```python
from build123d import *

# Parameters (mm, degrees)
F1_DEPTH = 5.08
F2_R     = 5.334
F2_R_2   = 2.54
F3_DEPTH = 2.54


with BuildPart() as f1:
    # F0 (on Front) → F1 (new body)
    with BuildSketch(Plane.XZ):
        with BuildLine():
            ThreePointArc((-33.39778, 15.875), (-36.091856, 14.759077), (-37.20778, 12.065))
            Line((-37.20778, 12.065), (-37.20778, 0))
            Line((-37.20778, 0), (-30.85778, 0))
            Line((-30.85778, 0), (-30.85778, 12.7))
            Line((-30.85778, 12.7), (-28.31778, 12.7))
            Line((-28.31778, 12.7), (-28.31778, 0))
            Line((-28.31778, 0), (-21.96778, 0))
            Line((-21.96778, 0), (-21.96778, 12.7))
            Line((-21.96778, 12.7), (-19.42778, 12.7))
            Line((-19.42778, 12.7), (-19.42778, 0))
            Line((-19.42778, 0), (-14.053237, 0))
            ThreePointArc((-14.053237, 0), (-11.513237, 2.54), (-8.973237, 0))
            Line((-8.973237, 0), (-3.893237, 0))
            ThreePointArc((-3.893237, 0), (-4.092609, 1.216333), (-4.669859, 2.305367))
            Line((-4.669859, 2.305367), (-13.839259, 14.370367))
            ThreePointArc((-13.839259, 14.370367), (-15.179614, 15.478177), (-16.872637, 15.875))
            Line((-16.872637, 15.875), (-33.39778, 15.875))
        make_face()
        with BuildLine():
            Line((-30.85778, 0), (-37.20778, 0))
            Line((-37.20778, 0), (-37.20778, -12.065))
            ThreePointArc((-37.20778, -12.065), (-36.091856, -14.759077), (-33.39778, -15.875))
            Line((-33.39778, -15.875), (-16.872637, -15.875))
            ThreePointArc((-16.872637, -15.875), (-15.179614, -15.478177), (-13.839259, -14.370367))
            Line((-13.839259, -14.370367), (-4.669859, -2.305367))
            ThreePointArc((-4.669859, -2.305367), (-4.092609, -1.216333), (-3.893237, 0))
            Line((-3.893237, 0), (-8.973237, 0))
            ThreePointArc((-8.973237, 0), (-11.513237, -2.54), (-14.053237, 0))
            Line((-14.053237, 0), (-19.42778, 0))
            Line((-19.42778, 0), (-19.42778, -12.7))
            Line((-19.42778, -12.7), (-21.96778, -12.7))
            Line((-21.96778, -12.7), (-21.96778, 0))
            Line((-21.96778, 0), (-28.31778, 0))
            Line((-28.31778, 0), (-28.31778, -12.7))
            Line((-28.31778, -12.7), (-30.85778, -12.7))
            Line((-30.85778, -12.7), (-30.85778, 0))
        make_face()
    extrude(amount=F1_DEPTH)

    # F2 (on face) → F3 (cut)
    with BuildSketch(Plane(origin=(0, 0, 0), x_dir=(-1, 0, 0), z_dir=(0, 1, 0))):
        with Locations((11.513237, 0)):
            Circle(F2_R)
        with Locations((11.513237, 0)):
            Circle(F2_R_2, mode=Mode.SUBTRACT)
    extrude(amount=-F3_DEPTH, mode=Mode.SUBTRACT)


solid = f1.part
```
Here's how the part is built. I have some questions about the finished solid (model axes, mm). A direction names the side the tool comes from. Give positions to 0.01 mm unless a question says otherwise; leave off trailing zeros. Loops run counter-clockwise (first coordinate to the right, second up) from the corner with the lowest first, then second, coordinate; pieces in that order, holes last. Notation, with made-up numbers: M 15.5,89.5 L 34.5,89.5 A25 ccw 34.5,108.5 Z; hole C -17,-9.5 d8. An arc over 180 degrees is marked long. Put each result on its own line as item: value. Start each with the question number.
(1) For faces 1 (the flat face through (-25, -3, 15.875)), 2 (the flat face through (-19.428, -3, 0)), 3 (the flat face through (-9, -2.54, -1)), which set-ups out of +Z, -Z, +X, -X, +Y, -Y let a thin tool reach every point of the face, with its end or its side?
(2) I need wall thicknesses on line 1 along Z through (x, y) = (-30.5, -1.4) (3 decimals); line 2 along X through (y, z) = (-2.5, -2.5); line 3 along X through (y, z) = (-3.6, -3). Which ranges of each line are inside material? Lowest first, please. Write a range as [from, to].
(3) I want a section at D-D on z = 11.5. Please give me the cut outline in (x, y).
(4) If we mould it in two halves opening along X, with no side actions, what happens to faces 4 (the flat face through (-24, 0, 0)), 5 (the cylindrical face through (-16.6, -1.3, 1.6)), 6 (the flat face through (-9, -3, 8))? For each: +X half, -X half, draft (parallel to the pull), parting line (faces both ways), or undercut.
(5) I want a section at A-A on y = -3.35. Please give me the cut outline in (x, z) (3 decimals).
(6) Will these pins go through, and if not, where does the flat tip stop? pin 1 Ø2 at (y, z) = (-2, 5.5) entering from +X; pin 2 Ø8 at (x, z) = (-11.51, 0) entering from +Y; pin 3 Ø1.5 at (y, z) = (-3, 12) entering from +X.
(7) I want a section at C-C on y = -1.2. Please give me the cut outline in (x, z) (3 decimals), then the cut area to 3 significant figures.
(8) I want a section at B-B on z = 6. Please give me the cut outline in (x, y).
Answer block:
1. face 1: +Z, +X, -X, +Y, -Y
1. face 2: +Y, -Y
1. face 3: +Y
2. line 1: [-15.875, -12.7], [12.7, 15.875]
2. line 2: [-37.21, -30.86], [-28.32, -21.97], [-19.43, -16.23], [-6.8, -4.82]
2. line 3: [-37.21, -30.86], [-28.32, -21.97], [-19.43, -5.2]
3. outline: M -37.21,-5.08 L -30.86,-5.08 L -30.86,0 L -37.21,0 Z; M -28.32,-5.08 L -21.97,-5.08 L -21.97,0 L -28.32,0 Z; M -19.43,-5.08 L -11.66,-5.08 L -11.66,0 L -19.43,0 Z
4. face 4: draft
4. face 5: undercut
4. face 6: +X half
5. outline: M -37.208,-12.065 A3.81 ccw -33.398,-15.875 L -16.873,-15.875 A3.81 ccw -13.839,-14.37 L -4.67,-2.305 A3.81 ccw -3.893,0 A3.81 ccw -4.67,2.305 L -13.839,14.37 A3.81 ccw -16.873,15.875 L -33.398,15.875 A3.81 ccw -37.208,12.065 Z; hole M -30.858,-12.7 L -28.318,-12.7 L -28.318,12.7 L -30.858,12.7 Z; hole M -21.968,-12.7 L -19.428,-12.7 L -19.428,12.7 L -21.968,12.7 Z; hole C -11.513,0 d5.08
6. pin 1: x = -6.34
6. pin 2: y = -2.54
6. pin 3: x = -11.47
7. outline: M -37.208,-12.065 A3.81 ccw -33.398,-15.875 L -16.873,-15.875 A3.81 ccw -13.839,-14.37 L -4.67,-2.305 A3.81 ccw -3.893,0 A3.81 ccw -4.67,2.305 L -13.839,14.37 A3.81 ccw -16.873,15.875 L -33.398,15.875 A3.81 ccw -37.208,12.065 Z; hole M -30.858,-12.7 L -28.318,-12.7 L -28.318,12.7 L -30.858,12.7 Z; hole M -21.968,-12.7 L -19.428,-12.7 L -19.428,12.7 L -21.968,12.7 Z; hole C -11.513,0 d10.668
7. area: 670 mm^2
8. outline: M -37.21,-5.08 L -30.86,-5.08 L -30.86,0 L -37.21,0 Z; M -28.32,-5.08 L -21.97,-5.08 L -21.97,0 L -28.32,0 Z; M -19.43,-5.08 L -7.48,-5.08 L -7.48,0 L -19.43,0 Z
